Autodesk Inventor part; units mm, degrees
ref_plane "YZ Plane" through (0, 0, 0) normal (1, 0, 0) x (0, 1, 0)
ref_plane "XZ Plane" through (0, 0, 0) normal (0, 1, 0) x (-1, 0, 0)
ref_plane "XY Plane" through (0, 0, 0) normal (0, 0, 1) x (1, 0, 0)
sketch "Sketch1" plane through (0, 0, 0) normal (1, 0, 0) x (0, 1, 0)
  line L0 (0, 0) -> (49.2107, 0)
  line L1 (49.2107, 0) -> (49.2107, -49.1998)
  line L2 (49.2107, -49.1998) -> (0, -49.1998)
  line L3 (0, -49.1998) -> (0, 0)
  circle A0 centre (28.5859, -28.575) radius 14.2748
  point P0 (42.8607, -28.575)
  point P1 (28.5859, -42.8498)
  dimension "d0" = 28.5859
  dimension "d1" = 28.5496
  dimension "d2" = 6.35
  dimension "d3" = 6.35
  dimension "d4" = 28.575
extrude "Extrusion1" add sketch "Sketch1" along normal blind 3.175
sketch "Sketch2" plane through (0, 0, -49.1998) normal (0, -1, 0) x (1, 0, 0)
  line L0 (3.175, 49.1998) -> (3.175, 0)
  line L1 (3.175, 49.1998) -> (15.875, 49.1998)
  line L2 (15.875, 49.1998) -> (15.875, 0)
  line L3 (15.875, 0) -> (3.175, 0)
  line L4 (3.175, 0) -> (3.175, 49.1998)
  point P0 (0, 49.1998)
  dimension "d7" = 12.7
extrude "Extrusion2" add sketch "Sketch2" along normal blind 3.175
sketch "Sketch3" plane through (0, 0, 0) normal (0, 0, 1) x (1, 0, 0)
  line L0 (3.175, 0) -> (3.175, 49.2107)
  line L1 (3.175, 0) -> (28.575, 0)
  line L2 (28.575, 0) -> (28.575, 49.2107)
  line L3 (28.575, 49.2107) -> (3.175, 49.2107)
  line L4 (3.175, 49.2107) -> (3.175, 0)
  point P0 (0, 0)
  dimension "d10" = 25.4
extrude "Extrusion3" add sketch "Sketch3" along normal blind 3.175
sketch "Sketch4" plane through (3.175, -3.175, 0) normal (0, 0, 1) x (1, 0, 0)
  line L0 (-3.175, 3.175) -> (0, 3.175)
  line L1 (0, 3.175) -> (0, 0)
  arc A0 (-3.175, 3.175) -> (0, 0) centre (0, 3.175) ccw
extrude "Extrusion4" add sketch "Sketch4" against normal up to surface (49.1998 mm away)
sketch "Sketch5" plane through (0, 49.2107, 0) normal (0, 1, 0) x (1, 0, 0)
  line L0 (3.175, 0) -> (3.175, -3.175)
  line L1 (0, 0) -> (3.175, 0)
  arc A0 (0, 0) -> (3.175, -3.175) centre (3.175, 0) ccw
extrude "Extrusion5" add sketch "Sketch5" against normal up to surface (49.2107 mm away)
sketch "Sketch6" plane through (0, 0, 3.175) normal (0, 0, 1) x (1, 0, 0)
  line L0 (3.175, 0) -> (28.575, 0)
  line L1 (28.575, 0) -> (28.575, 49.2107)
  line L2 (28.575, 49.2107) -> (3.175, 49.2107)
  line L3 (3.175, 49.2107) -> (3.175, 0)
  circle A0 centre (10.9643, 37.9241) radius 2.032
  circle A1 centre (20.7857, 37.9241) radius 2.032
  line L4 (12.9963, 37.9241) -> (18.7537, 37.9241)
  line L5 (8.9323, 37.9241) -> (3.175, 37.9241)
  line L6 (22.8177, 37.9241) -> (28.575, 37.9241)
  circle A2 centre (10.9643, 24.6054) radius 2.032
  circle A3 centre (10.9643, 11.2867) radius 2.032
  line L7 (10.9643, 39.9561) -> (10.9643, 49.2107)
  line L8 (28.575, 49.2107) -> (3.175, 49.2107)
  line L9 (10.9643, 26.6374) -> (10.9643, 35.8921)
  line L10 (10.9643, 13.3187) -> (10.9643, 22.5734)
  line L11 (10.9643, 9.2547) -> (10.9643, 0)
  circle A4 centre (20.7857, 24.6054) radius 2.032
  circle A5 centre (20.7857, 11.2867) radius 2.032
  point P0 (0, 0)
  dimension "d17" = 4.064
  dimension "d20" = 4.064
  dimension "d23" = 4.064
  dimension "d24" = 4.064
  dimension "d25" = 4.064
  dimension "d26" = 4.064
extrude "Extrusion6" cut sketch "Sketch6" against normal blind 3.175 contours A3 | A0 | A1 | A2 | A4 | A5
sketch "Sketch7" plane through (0, 0, -49.1998) normal (0, 1, 0) x (1, 0, 0)
  line L0 (3.175, -49.1998) -> (15.875, -49.1998)
  line L1 (15.875, -49.1998) -> (15.875, 0) construction
  line L2 (15.875, 0) -> (3.175, 0)
  line L3 (3.175, -49.1998) -> (3.175, 0)
  circle A0 centre (9.525, -11.284) radius 2.032
  circle A1 centre (9.525, -24.5999) radius 2.032
  circle A2 centre (9.525, -37.9158) radius 2.032
  line L4 (9.525, -9.2519) -> (9.525, 0)
  line L5 (9.525, -13.3159) -> (9.525, -22.5679) construction
  line L6 (9.525, -26.6319) -> (9.525, -35.8838)
  line L7 (9.525, -39.9478) -> (9.525, -49.1998)
  line L8 (28.575, -49.1998) -> (3.175, -49.1998)
  point P0 (0, -49.1998)
  dimension "d29" = 4.064
  dimension "d30" = 4.064
  dimension "d31" = 4.064
extrude "Extrusion7" cut sketch "Sketch7" against normal blind 3.175
properties part number "Robot to Bottomish Plate to Pivot Hex Axle"
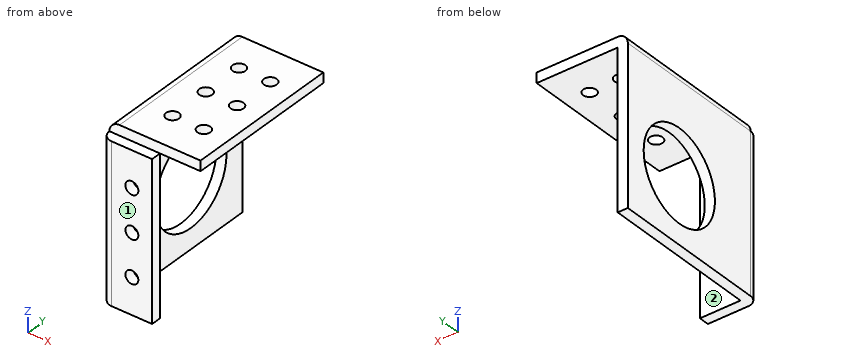
The model under review builds one solid part; all positions refer to its coordinate system, in mm. Face numbers are marked on the shaded views. A direction names the side the tool comes from. Round coordinates to 2 decimals unless told otherwise and drop trailing zeros. Order: outer loops, then holes, each group sorted by start corner. A loop starts at its lowest first (then second) coordinate and runs counter-clockwise, first axis right, second up. Notation, with made-up numbers: (68, 67.25) -> (109, 67.25) arc R30 cw to (109, 100.25) -> close; hole circle Ø6 at (9, 49). An arc over 180 degrees is marked (long way). Return JSON: item names as keys, results as strings.
1. For the marked faces 1 and 2, list the 3-axis set-ups (+Z, -Z, +X, -X, +Y, -Y) from which the entire face can be reached by the end or side of a thin tool; tool diameter is ignored.
Answer block:
{"face 1": "+Z, -Z, +X, -X, -Y", "face 2": "-Z, +X, +Y"}
2. Insertion check: P1, Ø12, axis at y = 8.5, z = -23.5, coming from the +X side (3 decimals); P2, Ø2.5, axis at x = 20.79, y = 37.92, coming from the +Z side; P3, Ø5.5, axis at x = 9.52, z = -24.6, coming from the +Y side; P4, Ø1.6, axis at x = 5, y = -2, coming from the +Z side. Each pin has a flat end and moves straight along its axis. Give the tip position at first contact, or say it passes through.
Answer block:
{"P1": "stops at x = 3.175", "P2": "passes through", "P3": "stops at y = 0", "P4": "stops at z = 0"}
3. For L1, parallel to Y at x = 13.75, z = -16.5 (3 decimals); L2, parallel to X at y = 12, z = -41.5 (3 decimals), list the stretches that pass through material, from the lowest coordinate up. Write a range as [from, to].
Answer block:
{"L1": "y = [-3.175, 0]", "L2": "x = [0, 3.175]"}
4. Take a section at B-B (y = 18.5). Write out the cut boundary in (x, z) (3 decimals), then the cut area to 3 significant figures.
Answer block:
{"outline": "(0, -49.2) -> (3.175, -49.2) -> (3.175, -38.677) -> (0, -38.677) -> close; (0, -18.473) -> (3.175, -18.473) -> (3.175, 0) -> (28.575, 0) -> (28.575, 3.175) -> (3.175, 3.175) arc R3.175 ccw to (0, 0) -> close", "area": "181 mm²"}
5. Take a section at C-C (z = -15). Write out the cut boundary in (x, y) (3 decimals), then the cut area to 3 significant figures.
Answer block:
{"outline": "(0, 0) arc R3.175 ccw to (3.175, -3.175) -> (15.875, -3.175) -> (15.875, 0) -> (3.175, 0) -> (3.175, 24.171) -> (0, 24.171) -> close; (0, 33.001) -> (3.175, 33.001) -> (3.175, 49.211) -> (0, 49.211) -> close", "area": "176 mm²"}
